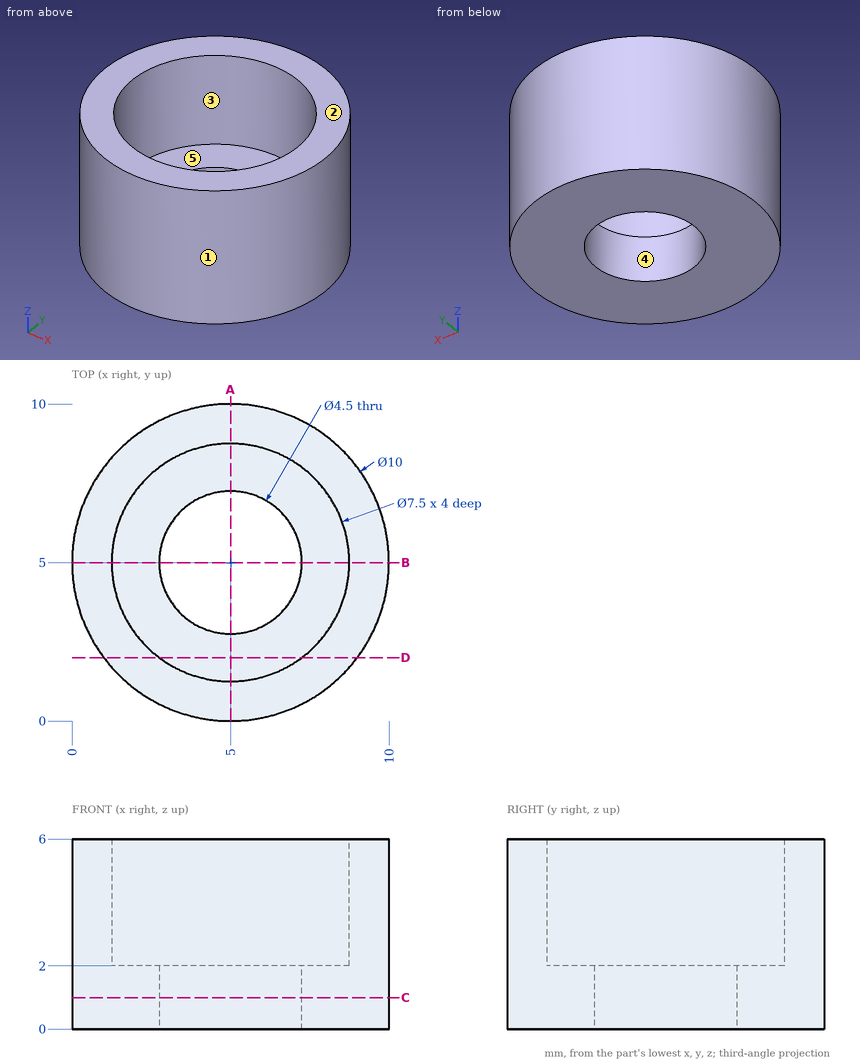
Geometry check sheet. Reference: drawing and pictorial views, mm from the part's lowest x, y, z. A direction names the side the tool comes from. Round coordinates to 2 decimals unless told otherwise and drop trailing zeros. Order: outer loops, then holes, each group sorted by start corner. A loop starts at its lowest first (then second) coordinate and runs counter-clockwise, first axis right, second up. Notation, with made-up numbers: M 45.5,37 L 54.5,37 A21 ccw 54.5,54 Z; hole C 56.25,5.5 d8. An arc over 180 degrees is marked long. One line per item, written item: value. Start each with the question number.
1. Section check A-A on x = 5. Enter the section's corners in (y, z).
2. Section check C-C on z = 1. Enter the section's corners in (x, y).
3. Section check D-D on y = 2. Enter the section's corners in (x, z), and give its area (3 significant figures).
4. Gauge pin test, flat ends, axial feed: P1, Ø1, axis at y = 6.5, z = 1, coming from the -X side; P2, Ø1, axis at x = 6, z = 1, coming from the -Y side; P3, Ø1.5, axis at x = 1.5, z = 2.5, coming from the -Y side. Record the tip position at first contact, or that the pin passes through.
5. Release check for a two-part mould opening along Y. For the marked faces 1, 2 and 3 record: released by +Y, released by -Y, zero draft, split by the parting line, or undercut.
6. Access from +Z, -Z, +X, -X, +Y, -Y to the whole of each face (thin tool, end or side, straight path). Record for the marked faces 4 and 5.
7. Scan lines: line 1 along Y through (x, z) = (5, 3.1); line 2 along Y through (x, z) = (5, 1.3); line 3 along Z through (x, y) = (2.5, 2.5). Record each from-to range of solid material in increasing order.
Results found:
1. outline: M 0,0 L 2.75,0 L 2.75,2 L 1.25,2 L 1.25,6 L 0,6 Z; M 7.25,0 L 10,0 L 10,6 L 8.75,6 L 8.75,2 L 7.25,2 Z
2. outline: C 5,5 d10; hole C 5,5 d4.5
3. outline: M 1,0 L 9,0 L 9,6 L 7.25,6 L 7.25,2 L 2.75,2 L 2.75,6 L 1,6 Z
3. area: 30.0 mm^2
4. P1: x = 0.1
4. P2: y = 0.03
4. P3: y = 0.82
5. face 1: split by the parting line
5. face 2: zero draft
5. face 3: undercut
6. face 4: +Z, -Z
6. face 5: +Z
7. line 1: 0 to 1.25, 8.75 to 10
7. line 2: 0 to 2.75, 7.25 to 10
7. line 3: 0 to 2
